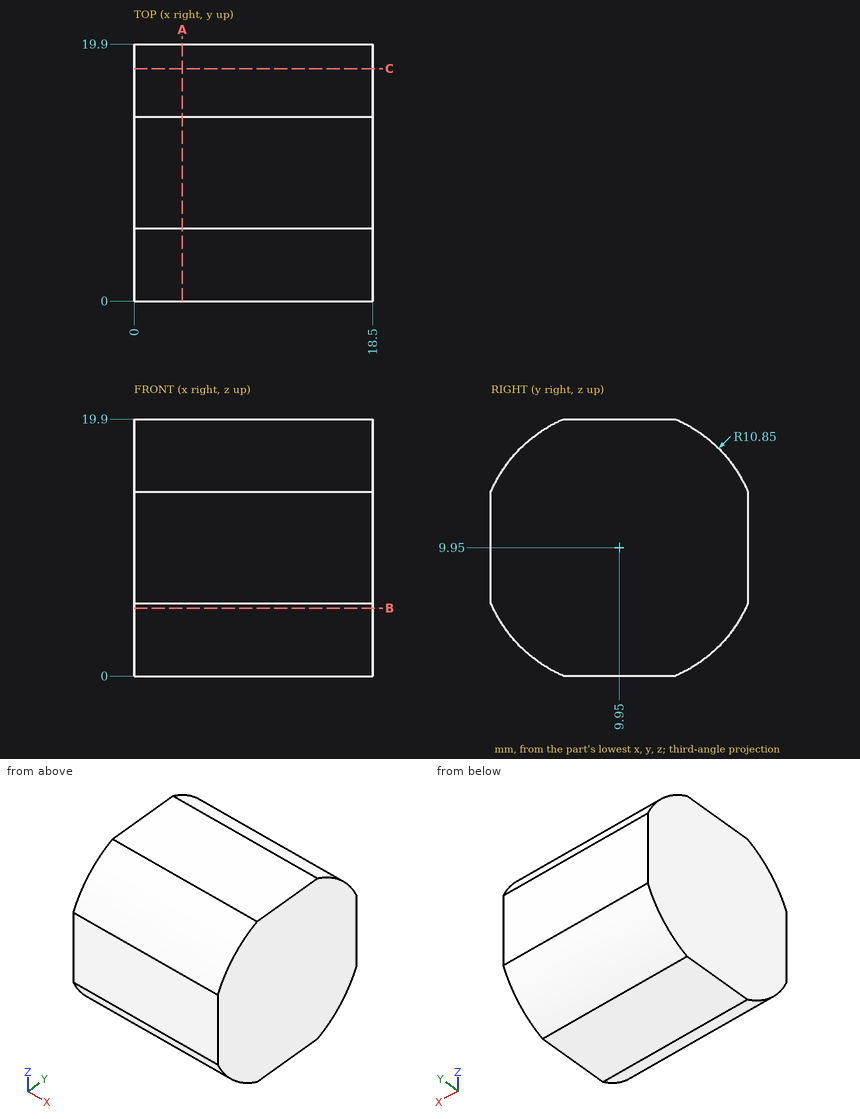
The drawing under review shows one solid part. Ordinate dimensions are in mm from its lowest x, y, z. Give positions to 0.01 mm unless a question says otherwise; leave off trailing zeros. Write each loop counter-clockwise with the first axis right and the second up, starting at its lowest first coordinate (ties: lowest second). Pieces come first, ordered by that corner, then holes.
1. Add section C-C, the plane y = 18. Write out the cut boundary in (x, z).
2. Add section B-B, the plane z = 5.25. Write out the cut boundary in (x, y).
3. Wall thickness on L1, parallel to Y at x = 12.5, z = 19; L2, parallel to Z at x = 9, y = 15.5; L3, parallel to Y at x = 12.25, z = 17.5: over which ranges is each line inside the solid? List them lowest first.
4. For P1, Ø4, axis at x = 15.5, y = 16.5, coming from the +Z side, flat-tipped, find the tip position at first contact; note if it passes through.
5. Add section A-A, the plane x = 3.75. Write out the cut boundary in (y, z).
Worked answers:
1. outline: (0, 2.68) - (18.5, 2.68) - (18.5, 17.22) - (0, 17.22) - close
2. outline: (0, 0.17) - (18.5, 0.17) - (18.5, 19.73) - (0, 19.73) - close
3. L1: y = 3.97 to 15.93
3. L2: z = 0.63 to 19.27
3. L3: y = 2.16 to 17.74
4. P1: stops at z = 19.8
5. outline: (0, 5.62) arc R10.85 ccw to (5.62, 0) - (14.28, 0) arc R10.85 ccw to (19.9, 5.62) - (19.9, 14.28) arc R10.85 ccw to (14.28, 19.9) - (5.62, 19.9) arc R10.85 ccw to (0, 14.28) - close
